Check sheet for the drawn part. Datum: minimum x, y, z corner. Units: mm. Coordinates: 2 decimals unless noted, no trailing zeros. Loops run counter-clockwise (first coordinate to the right, second up) from the corner with the lowest first, then second, coordinate; pieces in that order, holes last.
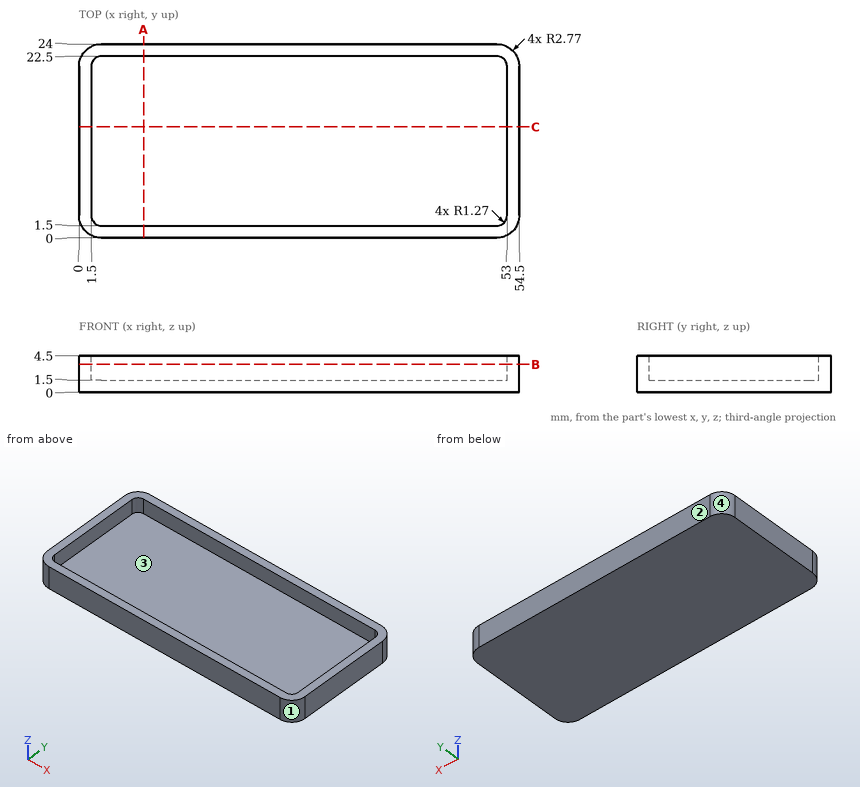
(1) Gauge pin test, flat ends, axial feed: pin 1 Ø6 at (x, y) = (32.5, 6.5) entering from +Z; pin 2 Ø5 at (x, y) = (28, 5.5) entering from -Z. Record the tip position at first contact, or that the pin passes through.
Findings:
pin 1: stops at z = 1.5
pin 2: stops at z = 0
(2) Scan lines: L1, parallel to Y at x = 39, z = 2.1; L2, parallel to X at y = 20.75, z = 2.8; L3, parallel to Z at x = 19.5, y = 5.5. Record each from-to range of solid material in increasing order.
Findings:
L1: y = 0 to 1.5, 22.5 to 24
L2: x = 0 to 1.5, 53 to 54.5
L3: z = 0 to 1.5
(3) Draft check along X on the marked faces 1, 2, 3 and 4. Enter one of: +X half, -X half, draft (parallel to the pull), parting line (faces both ways), or undercut.
Findings:
face 1: +X half
face 2: draft
face 3: undercut
face 4: -X half
(4) Sectioned sample at C-C on y = 13.75. Record the cut outline in (x, z).
Findings:
outline: (0, 0) - (54.5, 0) - (54.5, 4.5) - (53, 4.5) - (53, 1.5) - (1.5, 1.5) - (1.5, 4.5) - (0, 4.5) - close
(5) Sectioned sample at A-A on x = 8. Record the cut outline in (y, z).
Findings:
outline: (0, 0) - (24, 0) - (24, 4.5) - (22.5, 4.5) - (22.5, 1.5) - (1.5, 1.5) - (1.5, 4.5) - (0, 4.5) - close
(6) Sectioned sample at B-B on z = 3.45. Record the cut outline in (x, y).
Findings:
outline: (0, 2.77) arc R2.77 ccw to (2.77, 0) - (51.73, 0) arc R2.77 ccw to (54.5, 2.77) - (54.5, 21.23) arc R2.77 ccw to (51.73, 24) - (2.77, 24) arc R2.77 ccw to (0, 21.23) - close; hole (1.5, 2.77) arc R1.27 ccw to (2.77, 1.5) - (51.73, 1.5) arc R1.27 ccw to (53, 2.77) - (53, 21.23) arc R1.27 ccw to (51.73, 22.5) - (2.77, 22.5) arc R1.27 ccw to (1.5, 21.23) - close
